Geometry: final body of the model. Coordinates: model frame, mm. A direction names the side the tool comes from. Give positions to 0.01 mm unless a question says otherwise; leave off trailing zeros. Write each loop counter-clockwise with the first axis right and the second up, starting at its lowest first coordinate (ties: lowest second). Pieces come first, ordered by that corner, then holes. Notation, with made-up numbers: (-12.75, -24.75) - (-1.75, -24.75) arc R26 cw to (-1.75, -2.75) - close; hole circle Ø3 at (-35.5, -14). An arc over 180 degrees is marked (long way). Return JSON: item names as keys, results as strings.
from build123d import *

# Parameters (mm, degrees)
BOSS_EXTRUDE1_DEPTH = 2.75
SKETCH2_R           = 3.25
BOSS_EXTRUDE2_DEPTH = 20


# Read off the part's stored shape, not the designer's step: 1/4-20 Machine Threads Stud1
with BuildPart() as part:
    # Sketch1 → Boss-Extrude1 (new, symmetric)
    with BuildSketch(Plane.XY):
        Polygon((-9, 0), (-4.5, -7.794228634), (4.5, -7.794228634), (9, 0), (4.5, 7.794228634), (-4.5, 7.794228634), align=None)
    extrude(amount=BOSS_EXTRUDE1_DEPTH, both=True)

    # Sketch2 → Boss-Extrude2 (add)
    with BuildSketch(Plane.XY.offset(2.75)):
        Circle(SKETCH2_R)
    extrude(amount=BOSS_EXTRUDE2_DEPTH)

    # 1/4-20 Machine Threads Stud1 outline → 1/4-20 Machine Threads Stud1 (revolve, cut)
    with BuildSketch(Plane.XZ):
        Polygon((3.25, 22.75), (2.41935, 22.75), (3.175, 21.99435), (3.175, 7.75), (3.25, 7.75), align=None)
    revolve(axis=Axis((0, 0, 0), (0, 0, 1)), mode=Mode.SUBTRACT)


solid = part.part
Q1. Set-up query: faces 1 (the cylindrical face through (-2.579, -1.978, 5.215)), 2 (the flat face through (6.72, -3.95, 0.04)). Return all of +Z, -Z, +X, -X, +Y, -Y with unobstructed straight access to the full face (end or side cutting, diameter ignored); none if empty.
Answer key:
{"face 1": "+Z", "face 2": "+Z, -Z, +X, -Y"}
Q2. Section query A-A, the plane x = 0. Return the cut outline in (y, z) (3 decimals), plus the area to 3 significant figures.
Answer key:
{"outline": "(-7.794, -2.75) - (7.794, -2.75) - (7.794, 2.75) - (3.25, 2.75) - (3.25, 7.75) - (3.175, 7.75) - (3.175, 21.994) - (2.419, 22.75) - (-2.419, 22.75) - (-3.175, 21.994) - (-3.175, 7.75) - (-3.25, 7.75) - (-3.25, 2.75) - (-7.794, 2.75) - close", "area": "213 mm^2"}
Q3. Section query C-C, the plane y = 6.25. Return the cut outline in (x, z), plus the area to 3 significant figures.
Answer key:
{"outline": "(-5.39, -2.75) - (5.39, -2.75) - (5.39, 2.75) - (-5.39, 2.75) - close", "area": "59.3 mm^2"}
Q4. Pin query (flat end, axial travel): P1, Ø5, axis at x = 7, z = 6.5, coming from the +Y side; P2, Ø3, axis at x = 4, z = 5.5, coming from the -Y side. Return the tip coordinate at first contact, or that it passes through.
Answer key:
{"P1": "passes through", "P2": "stops at y = -2.08"}
Q5. Material intervals for probe 1 along Z at (x, y) = (-0.5, -7); probe 2 along Y at (x, z) = (-2.25, 14.75); probe 3 along X at (y, z) = (-2, 19.5), sorted ascending. Write a range as [from, to].
Answer key:
{"probe 1": "z = [-2.75, 2.75]", "probe 2": "y = [-2.24, 2.24]", "probe 3": "x = [-2.47, 2.47]"}
Q6. Section query B-B, the plane z = 11.5. Return the cut outline in (x, y) (3 decimals), plus the area to 3 significant figures.
Answer key:
{"outline": "circle Ø6.35 at (0, 0)", "area": "31.7 mm^2"}
